```python
from build123d import *

# Parameters (mm, degrees)
SKETCH1_R           = 22.5
BOSS_EXTRUDE4_DEPTH = 20
SKETCH1_6_R         = 22.5
BOSS_EXTRUDE5_DEPTH = 40


with BuildPart() as part:
    # Sketch1 → Boss-Extrude4 (new body)
    # profile 1 of 5: a face of its own
    with BuildSketch(Plane(origin=(0, 0, 0), x_dir=(1, 0, 0), z_dir=(0, 1, 0))):
        with BuildLine():
            ThreePointArc((4.941115981, -32.122194397), (24.666133355, -21.162038307), (32.5, 0))
            ThreePointArc((32.5, 0), (24.666133355, 21.162038307), (4.941115981, 32.122194397))
            ThreePointArc((4.941115981, 32.122194397), (-14.696219934, 28.987430373), (-28.831406487, 15))
            ThreePointArc((-28.831406487, 15), (-32.5, 0), (-28.831406487, -15))
            ThreePointArc((-28.831406487, -15), (-14.696219934, -28.987430373), (4.941115981, -32.122194397))
        make_face()
        with Locations(Location((0, 0, 0), (0, 0, 270))):
            Circle(SKETCH1_R, mode=Mode.SUBTRACT)
    # profile 2 of 5: a face of its own
    with BuildSketch(Plane(origin=(0, 0, 0), x_dir=(1, 0, 0), z_dir=(0, 1, 0))):
        with BuildLine():
            ThreePointArc((4.941115981, -32.122194397), (24.666133355, -21.162038307), (32.5, 0))
            ThreePointArc((32.5, 0), (24.666133355, 21.162038307), (4.941115981, 32.122194397))
            ThreePointArc((4.941115981, 32.122194397), (-14.696219934, 28.987430373), (-28.831406487, 15))
            ThreePointArc((-28.831406487, 15), (-32.5, 0), (-28.831406487, -15))
            ThreePointArc((-28.831406487, -15), (-14.696219934, -28.987430373), (4.941115981, -32.122194397))
        make_face()
        with Locations(Location((0, 0, 0), (0, 0, 270))):
            Circle(SKETCH1_R, mode=Mode.SUBTRACT)
    # profile 3 of 5: a face of its own
    with BuildSketch(Plane(origin=(0, 0, 0), x_dir=(1, 0, 0), z_dir=(0, 1, 0))):
        with BuildLine():
            ThreePointArc((60.5, 0), (62.696699141, 5.303300859), (68, 7.5))
            Line((68, 7.5), (100, 7.5))
            Line((100, 7.5), (100, 13.210304894))
            ThreePointArc((100, 13.210304894), (98.794789747, 16.466003095), (95.760171689, 18.152180955))
            Line((95.760171689, 18.152180955), (4.941115981, 32.122194397))
            ThreePointArc((4.941115981, 32.122194397), (24.666133355, 21.162038307), (32.5, 0))
            Line((32.5, 0), (60.5, 0))
        make_face()
    # profile 4 of 5: a face of its own
    with BuildSketch(Plane(origin=(0, 0, 0), x_dir=(1, 0, 0), z_dir=(0, 1, 0))):
        with BuildLine():
            ThreePointArc((68, -7.5), (62.696699141, -5.303300859), (60.5, 0))
            Line((60.5, 0), (32.5, 0))
            ThreePointArc((32.5, 0), (24.666133355, -21.162038307), (4.941115981, -32.122194397))
            Line((4.941115981, -32.122194397), (95.760171689, -18.152180955))
            ThreePointArc((95.760171689, -18.152180955), (98.794789747, -16.466003095), (100, -13.210304894))
            Line((100, -13.210304894), (100, -7.5))
            Line((100, -7.5), (68, -7.5))
        make_face()
    # profile 5 of 5: a face of its own
    with BuildSketch(Plane(origin=(0, 0, 0), x_dir=(1, 0, 0), z_dir=(0, 1, 0))):
        with BuildLine():
            ThreePointArc((-28.831406487, -15), (-32.5, 0), (-28.831406487, 15))
            Line((-28.831406487, 15), (-55, 15))
            Line((-55, 15), (-55, -15))
            Line((-55, -15), (-28.831406487, -15))
        make_face()
    extrude(amount=BOSS_EXTRUDE4_DEPTH)

    # Sketch1_6 → Boss-Extrude5 (add)
    # profile 1 of 2: a face of its own
    with BuildSketch(Plane(origin=(0, 0, 0), x_dir=(1, 0, 0), z_dir=(0, 1, 0))):
        with BuildLine():
            ThreePointArc((4.941115981, -32.122194397), (24.666133355, -21.162038307), (32.5, 0))
            ThreePointArc((32.5, 0), (24.666133355, 21.162038307), (4.941115981, 32.122194397))
            ThreePointArc((4.941115981, 32.122194397), (-14.696219934, 28.987430373), (-28.831406487, 15))
            ThreePointArc((-28.831406487, 15), (-32.5, 0), (-28.831406487, -15))
            ThreePointArc((-28.831406487, -15), (-14.696219934, -28.987430373), (4.941115981, -32.122194397))
        make_face()
        with Locations(Location((0, 0, 0), (0, 0, 270))):
            Circle(SKETCH1_6_R, mode=Mode.SUBTRACT)
    # profile 2 of 2: a face of its own
    with BuildSketch(Plane(origin=(0, 0, 0), x_dir=(1, 0, 0), z_dir=(0, 1, 0))):
        with BuildLine():
            ThreePointArc((4.941115981, -32.122194397), (24.666133355, -21.162038307), (32.5, 0))
            ThreePointArc((32.5, 0), (24.666133355, 21.162038307), (4.941115981, 32.122194397))
            ThreePointArc((4.941115981, 32.122194397), (-14.696219934, 28.987430373), (-28.831406487, 15))
            ThreePointArc((-28.831406487, 15), (-32.5, 0), (-28.831406487, -15))
            ThreePointArc((-28.831406487, -15), (-14.696219934, -28.987430373), (4.941115981, -32.122194397))
        make_face()
        with Locations(Location((0, 0, 0), (0, 0, 270))):
            Circle(SKETCH1_6_R, mode=Mode.SUBTRACT)
    extrude(amount=BOSS_EXTRUDE5_DEPTH)


solid = part.part
```
Verification items for the finished model (mm, model axes). A direction names the side the tool comes from. Coordinates: 2 decimals unless noted, no trailing zeros. Loops run counter-clockwise (first coordinate to the right, second up) from the corner with the lowest first, then second, coordinate; pieces in that order, holes last. Notation, with made-up numbers: (-24, -4.75) - (16, -4.75) arc R31 cw to (16, 26.25) - close; hole circle Ø2 at (37.25, 27). An arc over 180 degrees is marked (long way). Return JSON: item names as keys, results as strings.
1. Section check C-C, the plane z = 2. Record the boundary of the cut face in (x, y).
Established:
{"outline": "(-55, 0) - (-22.41, 0) - (-22.41, 40) - (-32.44, 40) - (-32.44, 20) - (-55, 20) - close; (22.41, 0) - (60.77, 0) - (60.77, 20) - (32.44, 20) - (32.44, 40) - (22.41, 40) - close"}
2. Section check A-A, the plane x = 0. Record the boundary of the cut face in (y, z), then the cut area to 3 significant figures.
Established:
{"outline": "(0, -32.5) - (40, -32.5) - (40, -22.5) - (0, -22.5) - close; (0, 22.5) - (40, 22.5) - (40, 32.5) - (0, 32.5) - close", "area": "800 mm2"}
3. Go/stop test with flat-tipped pins: pin 1 (6 mm diameter, centred on x = -39.5, y = 6.5, fed in from -Z); pin 2 (12 mm diameter, centred on y = 12, z = -20.5, fed in from +X); pin 3 (13 mm diameter, centred on x = -48, z = -1, fed in from +Y); pin 4 (12 mm diameter, centred on x = 40.5, z = 5.5, fed in from -Y). Record where each tip stops, or that it passes through.
Established:
{"pin 1": "stops at z = -15", "pin 2": "stops at x = 99.83", "pin 3": "stops at y = 20", "pin 4": "stops at y = 0"}
4. Section check B-B, the plane y = 18.5. Record the boundary of the cut face in (x, z), then the cut area to 3 significant figures.
Established:
{"outline": "(-55, -15) - (-28.83, -15) arc R32.5 ccw to (4.94, -32.12) - (95.76, -18.15) arc R5 ccw to (100, -13.21) - (100, -7.5) - (68, -7.5) arc R7.5 cw to (68, 7.5) - (100, 7.5) - (100, 13.21) arc R5 ccw to (95.76, 18.15) - (4.94, 32.12) arc R32.5 ccw to (-28.83, 15) - (-55, 15) - close; hole circle Ø45 at (0, 0)", "area": "5,240 mm2"}
5. Section check D-D, the plane z = -29. Record the boundary of the cut face in (x, y), then the cut area to 3 significant figures.
Established:
{"outline": "(-14.67, 0) - (25.24, 0) - (25.24, 20) - (14.67, 20) - (14.67, 40) - (-14.67, 40) - close", "area": "1,390 mm2"}
6. Thickness scan on L1, parallel to X at y = 15, z = 0; L2, parallel to Y at x = 45.5, z = 11; L3, parallel to X at y = 34, z = 17. Record the ranges inside material, lowest first.
Established:
{"L1": "x = -55 to -22.5, 22.5 to 60.5", "L2": "y = 0 to 20", "L3": "x = -27.7 to -14.74, 14.74 to 27.7"}
7. Mould release check, pull along Z, two halves, no side actions. Record for faces 5 (the flat face through (-55, 10, 0)), 6 (the flat face through (50.99, 9.86, -25.04)), 7 (the flat face through (84, 10, 7.5)): +Z half, -Z half, draft (parallel to the pull), parting line (faces both ways), or undercut.
Established:
{"face 5": "draft", "face 6": "-Z half", "face 7": "undercut"}
8. Tool access check on faces 1 (the flat face through (-42, 10, -15)), 2 (the flat face through (84, 10, -7.5)), 3 (the flat face through (-42, 10, 15)), 4 (the cylindrical face through (-32.43, 24.16, -2.14)). Record the directions out of +Z, -Z, +X, -X, +Y, -Y that give a thin tool (end or side, any length) a straight path to the whole face; none if there is none.
Established:
{"face 1": "-Z, -X, +Y, -Y", "face 2": "+X, +Y, -Y", "face 3": "+Z, -X, +Y, -Y", "face 4": "+Y"}
